Check sheet for the modelled part. Datum: model origin and axes. Units: mm. Face numbers are marked on the shaded views. Coordinates: 2 decimals unless noted, no trailing zeros. Order: outer loops, then holes, each group sorted by start corner. A loop starts at its lowest first (then second) coordinate and runs counter-clockwise, first axis right, second up. Notation, with made-up numbers: M 15,-30.75 L 56,-30.75 A17 ccw 56,-22.75 Z; hole C 59,7.25 d8. An arc over 180 degrees is marked long. Answer in a Markdown table with one row per item. Add a question column.
Autodesk Inventor part; units mm, degrees
ref_plane "YZ Plane" through (0, 0, 0) normal (1, 0, 0) x (0, 1, 0)
ref_plane "XZ Plane" through (0, 0, 0) normal (0, 1, 0) x (-1, 0, 0)
ref_plane "XY Plane" through (0, 0, 0) normal (0, 0, 1) x (1, 0, 0)
sketch "Sketch1" plane through (0, 0, 0) normal (0, 0, 1) x (1, 0, 0)
  line L0 (0, 0) -> (80, 0)
  line L1 (80, 0) -> (80, 25)
  line L2 (80, 25) -> (0, 25)
  line L3 (0, 25) -> (0, 0)
  point P0 (14.5, 19.7286)
  point P1 (14.5, 4.7286)
  point P2 (65.5, 19.7286)
  point P3 (65.5, 4.7286)
  dimension "d0" = 80
  dimension "d1" = 25
  dimension "d2" = 14.5
  dimension "d3" = 51
  dimension "d4" = 15
extrude "Extrusion1" add sketch "Sketch1" along normal blind 5
sketch "Sketch2" plane through (0, 0, 0) normal (0, 0, 1) x (1, 0, 0)
  line L0 (0, 0) -> (80, 0)
  line L1 (80, 0) -> (80, 25)
  line L2 (80, 25) -> (0, 25)
  line L3 (0, 25) -> (0, 0)
  point P0 (14.5, 19.7286)
  point P1 (14.5, 4.7286)
  point P2 (65.5, 19.7286)
  point P3 (65.5, 4.7286)
  dimension "d5" = 80
  dimension "d6" = 25
  dimension "d7" = 14.5
  dimension "d8" = 51
  dimension "d9" = 15
hole "Hole1" at (14.5, 19.7286, 0) at (14.5, 4.7286, 0) at (65.5, 19.7286, 0) at (65.5, 4.7286, 0) direction (0, 0, 1) diameter 3.5 end through all
sketch "Sketch3" plane through (0, 0, 5) normal (0, 0, 1) x (1, 0, 0)
  circle A0 centre (14.5, 19.7286) radius 1.75
  line L0 (16.25, 19.7286) -> (16.25, 4.7286)
  line L1 (12.75, 19.7286) -> (12.75, 4.7286)
  circle A1 centre (14.5, 4.7286) radius 1.75
  circle A2 centre (65.5, 19.7286) radius 1.75
  line L2 (63.75, 19.7286) -> (63.75, 4.7286)
  line L3 (67.25, 19.7286) -> (67.25, 4.7286)
  circle A3 centre (65.5, 4.7286) radius 1.75
  circle A4 centre (65.5, 19.7286) radius 1.75
  circle A5 centre (65.5, 4.7286) radius 1.75
  circle A6 centre (14.5, 19.7286) radius 1.75
  circle A7 centre (14.5, 4.7286) radius 1.75
  point P0 (0, 0)
extrude "Extrusion2" cut sketch "Sketch3" against normal blind 5 contours L0 A1 L1 A0 | L3 A3 L2 A2
fillet "Fillet1" radius 2 4 edges at (80, 25, 2.5) (80, 0, 2.5) (0, 25, 2.5) (0, 0, 2.5)
sketch "Sketch4" plane through (0, 0, 5) normal (0, 0, 1) x (1, 0, 0)
  line L0 (63.75, 4.7286) -> (63.75, 19.7286)
  arc A0 (67.25, 19.7286) -> (63.75, 19.7286) centre (65.5, 19.7286) ccw
  line L1 (67.25, 19.7286) -> (67.25, 4.7286)
  arc A1 (63.75, 4.7286) -> (67.25, 4.7286) centre (65.5, 4.7286) ccw
  line L2 (12.75, 4.7286) -> (12.75, 19.7286)
  arc A2 (16.25, 19.7286) -> (12.75, 19.7286) centre (14.5, 19.7286) ccw
  line L3 (16.25, 19.7286) -> (16.25, 4.7286)
  arc A3 (12.75, 4.7286) -> (16.25, 4.7286) centre (14.5, 4.7286) ccw
  arc A4 (0, 2) -> (2, 0) centre (2, 2) ccw
  line L4 (2, 0) -> (78, 0)
  arc A5 (78, 0) -> (80, 2) centre (78, 2) ccw
  line L5 (80, 2) -> (80, 23)
  arc A6 (80, 23) -> (78, 25) centre (78, 23) ccw
  line L6 (78, 25) -> (2, 25)
  arc A7 (2, 25) -> (0, 23) centre (2, 23) ccw
  line L7 (0, 23) -> (0, 2)
  point P0 (0, 0)
properties part number "BasePatasVTOL2"
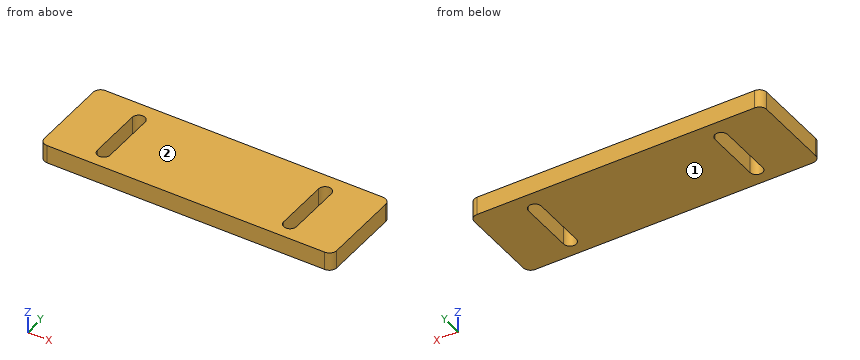
1. Section check A-A on y = 18. Enter the section's corners in (x, z).
2. Scan lines: line 1 (X direction, y = 7.75, z = 4.3); line 2 (X direction, y = 3.75, z = 3); line 3 (X direction, y = 23.5, z = 2.8). Record each from-to range of solid material in increasing order.
3. Section check B-B on z = 1.9. Enter the section's corners in (x, y), then the cut area to 3 significant figures.
4. Release check for a two-part mould opening along Z. For the marked faces 1 and 2 record: released by +Z, released by -Z, zero draft, split by the parting line, or undercut.
5. Section check C-C on x = 14.5. Enter the section's corners in (y, z).
Result sheet:
| question | item | result |
|---|---|---|
| 1 | outline | M 0,0 L 12.75,0 L 12.75,5 L 0,5 Z; M 16.25,0 L 63.75,0 L 63.75,5 L 16.25,5 Z; M 67.25,0 L 80,0 L 80,5 L 67.25,5 Z |
| 2 | line 1 | 0 to 12.75, 16.25 to 63.75, 67.25 to 80 |
| 2 | line 2 | 0 to 13.05, 15.95 to 64.05, 66.95 to 80 |
| 2 | line 3 | 0.06 to 79.94 |
| 3 | outline | M 0,2 A2 ccw 2,0 L 78,0 A2 ccw 80,2 L 80,23 A2 ccw 78,25 L 2,25 A2 ccw 0,23 Z; hole M 12.75,4.73 A1.75 ccw 16.25,4.73 L 16.25,19.73 A1.75 ccw 12.75,19.73 Z; hole M 63.75,4.73 A1.75 ccw 67.25,4.73 L 67.25,19.73 A1.75 ccw 63.75,19.73 Z |
| 3 | area | 1,870 mm^2 |
| 4 | face 1 | released by -Z |
| 4 | face 2 | released by +Z |
| 5 | outline | M 0,0 L 2.98,0 L 2.98,5 L 0,5 Z; M 21.48,0 L 25,0 L 25,5 L 21.48,5 Z |
